Model file for the job. Use its own axes, mm. Face numbers are marked on the shaded views. A direction names the side the tool comes from. Round coordinates to 2 decimals unless told otherwise and drop trailing zeros. Order: outer loops, then holes, each group sorted by start corner. A loop starts at its lowest first (then second) coordinate and runs counter-clockwise, first axis right, second up. Notation, with made-up numbers: (9.5, 56.25) -> (53.5, 56.25) arc R17 ccw to (53.5, 84.25) -> close; hole circle Ø10 at (-22.75, 36.5). An arc over 180 degrees is marked (long way). Answer as CSV lines item,"result".
```python
from build123d import *

# Parameters (mm, degrees)
SKETCH_1_W        = 66
SKETCH_1_H        = 66
EXTRUDE_1_DEPTH   = 3
SKETCH_1_2_W      = 72
SKETCH_1_2_H      = 72
SKETCH_1_2_W_2    = 66
SKETCH_1_2_H_2    = 66
EXTRUDE_1_2_DEPTH = 25
FILLET_1_R        = 2


with BuildPart() as part:
    # 草图1 → Extrude 1 (new body)
    with BuildSketch(Plane(origin=(0, 0, 0), x_dir=(1, 0, 0), z_dir=(0, 1, 0))):
        Rectangle(SKETCH_1_W, SKETCH_1_H)
    extrude(amount=EXTRUDE_1_DEPTH)

    # 草图1<2> → Extrude 1 2 (add)
    with BuildSketch(Plane(origin=(0, 0, 0), x_dir=(1, 0, 0), z_dir=(0, 1, 0))):
        Rectangle(SKETCH_1_2_W, SKETCH_1_2_H)
        Rectangle(SKETCH_1_2_W_2, SKETCH_1_2_H_2, mode=Mode.SUBTRACT)
    extrude(amount=EXTRUDE_1_2_DEPTH)

    # 圆角1
    fillet_1_edges = [part.edges().sort_by_distance(p)[0] for p in [
        (36, 0, 0),
        (36, 12.5, 36),
        (0, 0, -36),
        (36, 12.5, -36),
        (-36, 0, 0),
        (-36, 12.5, -36),
        (0, 0, 36),
        (-36, 12.5, 36),
    ]]
    fillet(fillet_1_edges, radius=FILLET_1_R)


solid = part.part
```
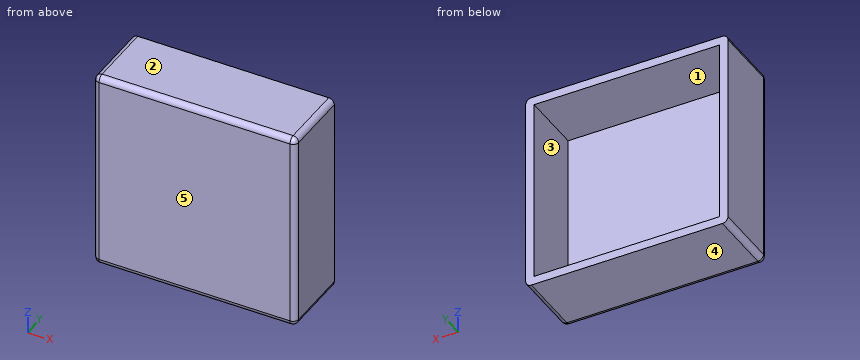
Q1. Mould opens along Z. For the marked faces 3, 4 and 5 say: +Z half, -Z half, draft (parallel to the pull), parting line (faces both ways), or undercut.
Checks:
face 3,"undercut"
face 4,"-Z half"
face 5,"draft"
Q2. Saw through at C-C (y = 9.5). Write the cut outline in (x, z), plus the area to 3 significant figures.
Checks:
outline,"(-36, -34) arc R2 ccw to (-34, -36) -> (34, -36) arc R2 ccw to (36, -34) -> (36, 34) arc R2 ccw to (34, 36) -> (-34, 36) arc R2 ccw to (-36, 34) -> close; hole (-33, -33) -> (33, -33) -> (33, 33) -> (-33, 33) -> close"
area,"825 mm²"
Q3. Saw through at B-B (z = 26). Write the cut outline in (x, y).
Checks:
outline,"(-36, 2) arc R2 ccw to (-34, 0) -> (34, 0) arc R2 ccw to (36, 2) -> (36, 25) -> (33, 25) -> (33, 3) -> (-33, 3) -> (-33, 25) -> (-36, 25) -> close"
Q4. Wall check: L1, parallel to X at y = 8, z = 22; L2, parallel to Y at x = -15, z = 23. Give the ranges that are in metal, low to high. Write a range as [from, to].
Checks:
L1,"[-36, -33], [33, 36]"
L2,"[0, 3]"
Q5. Tool access for the marked faces 1 and 2: list every direction of +Z, -Z, +X, -X, +Y, -Y with a clear straight run to the whole face (end or side of a thin tool).
Checks:
face 1,"+Y"
face 2,"+Z, +X, -X, +Y, -Y"
Q6. Flat gauge pin, fed straight in: pin 1 (20 mm diameter, centred on x = 11.5, z = -5.5, fed in from +Y). Where does the tip first touch, or does it go through?
Checks:
pin 1,"y = 3"
Q7. Saw through at A-A (x = 7). Write the cut outline in (y, z).
Checks:
outline,"(0, -34) arc R2 ccw to (2, -36) -> (25, -36) -> (25, -33) -> (3, -33) -> (3, 33) -> (25, 33) -> (25, 36) -> (2, 36) arc R2 ccw to (0, 34) -> close"
